For this review, take the finished solid that the model builds, in its own axes (mm). A direction names the side the tool comes from. Give positions to 0.01 mm unless a question says otherwise; leave off trailing zeros. Order: outer loops, then holes, each group sorted by start corner. A loop starts at its lowest first (then second) coordinate and runs counter-clockwise, first axis right, second up. Notation, with made-up numbers: (59, 25.5) -> (71, 25.5) arc R23 ccw to (71, 41.5) -> close; hole circle Ø9 at (72, 41). An arc over 180 degrees is marked (long way). Return JSON: item names as keys, results as strings. Group by question number.
1) Add section B-B (z = -4). Give the boundary of the cut face in (x, y).
2) To check wall thickness, follow line 1 along X through (y, z) = (17.5, -2); line 2 along X through (y, z) = (-12.5, 27.5); line 3 along Z through (x, y) = (10.5, 6). State the ranges of each line that lie inside material, in increasing order.
3) Add section C-C (x = 68.5). Give the boundary of the cut face in (y, z).
4) Add section A-A (y = 10). Give the boundary of the cut face in (x, z).
5) Insertion check: P1, Ø6.5, axis at y = 19.5, z = 28.5, coming from the -X side; P2, Ø1, axis at x = -1, z = 40, coming from the -Y side (3 decimals); P3, Ø18.5, axis at y = 8, z = 10.5, coming from the +X side; P4, Ø24.5, axis at x = 65, z = 41, coming from the -Y side. Each pin has a flat end and moves straight along its axis. Give the tip position at first contact, or say it passes through.
6) For faces 1 (the face through (40.15, 14.13, 75.72)), 2 (the face through (1, -34, 11.303)), 3 (the face through (71, 0, 66.837)), 4 (the face through (48, 25.4, 49)), list the 3-axis set-ups (+Z, -Z, +X, -X, +Y, -Y) from which the entire face can be reached by the end or side of a thin tool; tool diameter is ignored.
from build123d import *

# Parameters (mm, degrees)
F1_DEPTH = 63.5
F2_DEPTH = 25.4
F3_DEPTH = 3.175


with BuildPart() as f1:
    # F0 (on Front) → F1 (new body, symmetric)
    with BuildSketch(Plane.XZ):
        Polygon((-48.475966, -11.303), (48.475966, -11.303), (48.475966, 11.303), (29.425966, 11.303), (-48.475966, 11.303), align=None)
    extrude(amount=F1_DEPTH, both=True)

    # F0 (on Front) → F2 (join, symmetric)
    with BuildSketch(Plane.XZ):
        with BuildLine():
            Line((29.425966, 11.303), (48.475966, 11.303))
            Line((48.475966, 11.303), (48.475966, 50.224972))
            ThreePointArc((48.475966, 50.224972), (53.341391, 61.971147), (65.087566, 66.836572))
            Line((65.087566, 66.836572), (77.961333, 66.836572))
            Line((77.961333, 66.836572), (77.961333, 85.886572))
            Line((77.961333, 85.886572), (65.087566, 85.886572))
            ThreePointArc((65.087566, 85.886572), (39.871007, 75.441531), (29.425966, 50.224972))
            Line((29.425966, 50.224972), (29.425966, 11.303))
        make_face()
    extrude(amount=F2_DEPTH, both=True)

    # F0 (on Front) → F3 (join, symmetric)
    with BuildSketch(Plane.XZ):
        with BuildLine():
            add(Edge.make_bspline(
                [(-48.475966, 11.303), (-36.481909, 55.469651), (13.493313, 85.954547), (65.087566, 85.886572)],
                knots=[0, 0, 0, 0, 135.865319, 135.865319, 135.865319, 135.865319], degree=3))
            Line((-48.475966, 11.303), (29.425966, 11.303))
            Line((29.425966, 11.303), (29.425966, 50.224972))
            ThreePointArc((29.425966, 50.224972), (39.871007, 75.441531), (65.087566, 85.886572))
        make_face()
    extrude(amount=F3_DEPTH, both=True)


solid = f1.part
Evaluation:
{
 "1": {"outline": "(-48.48, -63.5) -> (48.48, -63.5) -> (48.48, 63.5) -> (-48.48, 63.5) -> close"},
 "2": {"line 1": "-48.48 to 48.48", "line 2": "29.43 to 48.48", "line 3": "-11.3 to 11.3"},
 "3": {"outline": "(-25.4, 66.84) -> (25.4, 66.84) -> (25.4, 85.89) -> (-25.4, 85.89) -> close"},
 "4": {"outline": "(-48.48, -11.3) -> (48.48, -11.3) -> (48.48, 50.22) arc R16.61 cw to (65.09, 66.84) -> (77.96, 66.84) -> (77.96, 85.89) -> (65.09, 85.89) arc R35.66 ccw to (29.43, 50.22) -> (29.43, 11.3) -> (-48.48, 11.3) -> close"},
 "5": {"P1": "x = 29.43", "P2": "y = -3.175", "P3": "x = 48.48", "P4": "through"},
 "6": {"face 1": "+Z, -X, +Y", "face 2": "+Z, -X, -Y", "face 3": "-Z, +X, +Y, -Y", "face 4": "+Z, +X, -X, +Y"}
}
